from build123d import *

# Parameters (mm, degrees)
F1_DEPTH = 2
F2_DEPTH = 5


with BuildPart() as f1:
    # F0 (on Top) → F1 (new body)
    with BuildSketch(Plane.XY):
        with BuildLine():
            Line((-21.71096, -0.986954), (-6.21096, -0.986954))
            ThreePointArc((-6.21096, -0.986954), (0.860108, 1.941978), (3.78904, 9.013046))
            Line((3.78904, 9.013046), (3.78904, 29.513046))
            ThreePointArc((3.78904, 29.513046), (0.860108, 36.584114), (-6.21096, 39.513046))
            Line((-6.21096, 39.513046), (-21.71096, 39.513046))
            ThreePointArc((-21.71096, 39.513046), (-28.782028, 36.584114), (-31.71096, 29.513046))
            Line((-31.71096, 29.513046), (-31.71096, 9.013046))
            ThreePointArc((-31.71096, 9.013046), (-28.782028, 1.941978), (-21.71096, -0.986954))
        make_face()
        with BuildLine():
            ThreePointArc((1.78904, 9.013046), (-0.554106, 3.356191), (-6.21096, 1.013046))
            Line((-6.21096, 1.013046), (-21.71096, 1.013046))
            ThreePointArc((-21.71096, 1.013046), (-27.367814, 3.356191), (-29.71096, 9.013046))
            Line((-29.71096, 9.013046), (-29.71096, 29.513046))
            ThreePointArc((-29.71096, 29.513046), (-27.367814, 35.1699), (-21.71096, 37.513046))
            Line((-21.71096, 37.513046), (-6.21096, 37.513046))
            ThreePointArc((-6.21096, 37.513046), (-0.554106, 35.1699), (1.78904, 29.513046))
            Line((1.78904, 29.513046), (1.78904, 9.013046))
        make_face(mode=Mode.SUBTRACT)
        with BuildLine():
            Line((-21.71096, 1.013046), (-6.21096, 1.013046))
            ThreePointArc((-6.21096, 1.013046), (-0.554106, 3.356191), (1.78904, 9.013046))
            Line((1.78904, 9.013046), (1.78904, 29.513046))
            ThreePointArc((1.78904, 29.513046), (-0.554106, 35.1699), (-6.21096, 37.513046))
            Line((-6.21096, 37.513046), (-21.71096, 37.513046))
            ThreePointArc((-21.71096, 37.513046), (-27.367814, 35.1699), (-29.71096, 29.513046))
            Line((-29.71096, 29.513046), (-29.71096, 9.013046))
            ThreePointArc((-29.71096, 9.013046), (-27.367814, 3.356191), (-21.71096, 1.013046))
        make_face()
    extrude(amount=F1_DEPTH)

    # F0 (on Top) → F2 (join)
    with BuildSketch(Plane.XY):
        with BuildLine():
            Line((-21.71096, -0.986954), (-6.21096, -0.986954))
            ThreePointArc((-6.21096, -0.986954), (0.860108, 1.941978), (3.78904, 9.013046))
            Line((3.78904, 9.013046), (3.78904, 29.513046))
            ThreePointArc((3.78904, 29.513046), (0.860108, 36.584114), (-6.21096, 39.513046))
            Line((-6.21096, 39.513046), (-21.71096, 39.513046))
            ThreePointArc((-21.71096, 39.513046), (-28.782028, 36.584114), (-31.71096, 29.513046))
            Line((-31.71096, 29.513046), (-31.71096, 9.013046))
            ThreePointArc((-31.71096, 9.013046), (-28.782028, 1.941978), (-21.71096, -0.986954))
        make_face()
        with BuildLine():
            ThreePointArc((1.78904, 9.013046), (-0.554106, 3.356191), (-6.21096, 1.013046))
            Line((-6.21096, 1.013046), (-21.71096, 1.013046))
            ThreePointArc((-21.71096, 1.013046), (-27.367814, 3.356191), (-29.71096, 9.013046))
            Line((-29.71096, 9.013046), (-29.71096, 29.513046))
            ThreePointArc((-29.71096, 29.513046), (-27.367814, 35.1699), (-21.71096, 37.513046))
            Line((-21.71096, 37.513046), (-6.21096, 37.513046))
            ThreePointArc((-6.21096, 37.513046), (-0.554106, 35.1699), (1.78904, 29.513046))
            Line((1.78904, 29.513046), (1.78904, 9.013046))
        make_face(mode=Mode.SUBTRACT)
    extrude(amount=F2_DEPTH)


solid = f1.part
Geometry check sheet. Reference: the model listing, model coordinates, mm. A direction names the side the tool comes from. Coordinates: 2 decimals unless noted, no trailing zeros. Order: outer loops, then holes, each group sorted by start corner. A loop starts at its lowest first (then second) coordinate and runs counter-clockwise, first axis right, second up. Notation, with made-up numbers: (-25.5, -19.5) -> (26.5, -19.5) arc R16 cw to (26.5, 4.5) -> close; hole circle Ø10 at (-30, 89). An arc over 180 degrees is marked (long way). Use a Markdown table: item, result. Add a question column.
1. Material ranges on L1, parallel to Y at x = -11, z = 4; L2, parallel to X at y = 24, z = 2.65; L3, parallel to Z at x = -25, y = 13, recorded low to high.
2. Mould release check, pull along Y, two halves, no side actions. Record for faces 3 (the face through (-28.86, 2.02, 2.46)), 4 (the face through (-27.43, 35.107, 3.479)), 5 (the face through (-28.704, 36.661, 2.465)), 6 (the face through (-0.617, 35.232, 3.479)): pulls with the +Y half, pulls with the -Y half, needs draft (parallel to the pull), parting line crosses it, or undercut.
3. Cross-section at C-C (y = 19.5). Enter the section's corners in (x, z), and give its area (3 significant figures).
4. Go/stop test with a flat-tipped pin: pin 1 Ø3 at (x, y) = (-25.5, 17) entering from +Z. Record where the tip stops, or that it passes through.
5. Cross-section at B-B (x = -11.5). Enter the section's corners in (y, z).
6. Set-up check for faces 1 (the face through (1.789, 19, 3)), 2 (the face through (-30, 19, 5)): record each of +Z, -Z, +X, -X, +Y, -Y from which the full face is reachable in a straight line by a thin tool's end or side.
7. Cross-section at A-A (z = 2.75). Enter the section's corners in (x, y), and give its area (3 significant figures).
Filled sheet:
| question | item | result |
|---|---|---|
| 1 | L1 | -0.99 to 1.01, 37.51 to 39.51 |
| 1 | L2 | -31.71 to -29.71, 1.79 to 3.79 |
| 1 | L3 | 0 to 2 |
| 2 | face 3 | pulls with the -Y half |
| 2 | face 4 | undercut |
| 2 | face 5 | pulls with the +Y half |
| 2 | face 6 | undercut |
| 3 | outline | (-31.71, 0) -> (3.79, 0) -> (3.79, 5) -> (1.79, 5) -> (1.79, 2) -> (-29.71, 2) -> (-29.71, 5) -> (-31.71, 5) -> close |
| 3 | area | 83.0 mm2 |
| 4 | pin 1 | z = 2 |
| 5 | outline | (-0.99, 0) -> (39.51, 0) -> (39.51, 5) -> (37.51, 5) -> (37.51, 2) -> (1.01, 2) -> (1.01, 5) -> (-0.99, 5) -> close |
| 6 | face 1 | +Z |
| 6 | face 2 | +Z, +X, -X, +Y, -Y |
| 7 | outline | (-31.71, 9.01) arc R10 ccw to (-21.71, -0.99) -> (-6.21, -0.99) arc R10 ccw to (3.79, 9.01) -> (3.79, 29.51) arc R10 ccw to (-6.21, 39.51) -> (-21.71, 39.51) arc R10 ccw to (-31.71, 29.51) -> close; hole (-29.71, 9.01) arc R8 ccw to (-21.71, 1.01) -> (-6.21, 1.01) arc R8 ccw to (1.79, 9.01) -> (1.79, 29.51) arc R8 ccw to (-6.21, 37.51) -> (-21.71, 37.51) arc R8 ccw to (-29.71, 29.51) -> close |
| 7 | area | 257 mm2 |
